Work out the finished part from the listing and answer in its coordinate system (mm). A direction names the side the tool comes from. Give positions to 0.01 mm unless a question says otherwise; leave off trailing zeros. Loops run counter-clockwise (first coordinate to the right, second up) from the corner with the lowest first, then second, coordinate; pieces in that order, holes last. Notation, with made-up numbers: M -1,41 L 20,41 A31 cw 20,73 Z; hole C -37,50.25 d7. An arc over 180 degrees is marked long. Answer as a JSON object with one key per item and string values. Group by question number.
```python
from build123d import *

# Parameters (mm, degrees)
SKETCH_1_R      = 1.5
EXTRUDE_1_DEPTH = 1.5
SKETCH_2_W      = 10
SKETCH_2_H      = 7.5
EXTRUDE_2_DEPTH = 10
SKETCH_3_W      = 8
SKETCH_3_H      = 8
EXTRUDE_3_DEPTH = 8
SKETCH_4_W      = 15
SKETCH_4_H      = 7.5
EXTRUDE_4_DEPTH = 10
EXTRUDE_5_DEPTH = 25
SKETCH_6_W      = 4
SKETCH_6_H      = 4
EXTRUDE_6_DEPTH = 4
SKETCH_7_W      = 20
SKETCH_7_H      = 5
EXTRUDE_7_DEPTH = 14
SKETCH_8_W      = 12
SKETCH_8_H      = 12
SKETCH_8_W_2    = 10
SKETCH_8_H_2    = 8
EXTRUDE_8_DEPTH = 8
SKETCH_9_R      = 4
EXTRUDE_9_DEPTH = 10


with BuildPart() as part:
    # 草图1 → 凸台-拉伸1 (new body)
    with BuildSketch(Plane(origin=(0, 0, 0), x_dir=(1, 0, 0), z_dir=(0, 1, 0))):
        with BuildLine():
            Line((-41.7, 30), (41.7, 30))
            ThreePointArc((41.7, 30), (44.033452378, 29.033452378), (45, 26.7))
            Line((45, 26.7), (45, -26.7))
            ThreePointArc((45, -26.7), (44.033452378, -29.033452378), (41.7, -30))
            Line((41.7, -30), (-41.7, -30))
            ThreePointArc((-41.7, -30), (-44.033452378, -29.033452378), (-45, -26.7))
            Line((-45, -26.7), (-45, 26.7))
            ThreePointArc((-45, 26.7), (-44.033452378, 29.033452378), (-41.7, 30))
        make_face()
        with Locations((-41.35, 26.4)):
            Circle(SKETCH_1_R, mode=Mode.SUBTRACT)
        with Locations((41.35, 26.4)):
            Circle(SKETCH_1_R, mode=Mode.SUBTRACT)
        with Locations((41.35, -26.4)):
            Circle(SKETCH_1_R, mode=Mode.SUBTRACT)
        with Locations((-41.35, -26.4)):
            Circle(SKETCH_1_R, mode=Mode.SUBTRACT)
    extrude(amount=EXTRUDE_1_DEPTH)

    # 草图2 → 凸台-拉伸2 (add)
    with BuildSketch(Plane(origin=(0, 1.5, 0), x_dir=(1, 0, 0), z_dir=(0, 1, 0))):
        with Locations((18.5, -23.75)):
            Rectangle(SKETCH_2_W, SKETCH_2_H)
        with Locations((-9.5, 23.75)):
            Rectangle(SKETCH_2_W, SKETCH_2_H)
        with Locations((9.5, 23.75)):
            Rectangle(SKETCH_2_W, SKETCH_2_H)
        with Locations((-18.5, -23.75)):
            Rectangle(SKETCH_2_W, SKETCH_2_H)
    extrude(amount=EXTRUDE_2_DEPTH)

    # 草图3 → 凸台-拉伸3 (add)
    with BuildSketch(Plane(origin=(0, 1.5, 0), x_dir=(1, 0, 0), z_dir=(0, 1, 0))):
        with Locations((-8.2, -23.75)):
            Rectangle(SKETCH_3_W, SKETCH_3_H)
    extrude(amount=EXTRUDE_3_DEPTH)

    # 草图4 → 凸台-拉伸4 (add)
    with BuildSketch(Plane(origin=(0, 1.5, 0), x_dir=(1, 0, 0), z_dir=(0, 1, 0))):
        with Locations((4.7, -23.75)):
            Rectangle(SKETCH_4_W, SKETCH_4_H)
    extrude(amount=EXTRUDE_4_DEPTH)

    # 草图5 → 凸台-拉伸5 (add)
    with BuildSketch(Plane(origin=(0, 1.5, 0), x_dir=(1, 0, 0), z_dir=(0, 1, 0))):
        Polygon((44.8, 16), (28.8, 16), (28.8, 15.4), (36.2, 15.4), (36.2, -6.4), (28.8, -6.4), (28.8, -7), (44.8, -7), (44.8, -6.4), (36.8, -6.4), (36.8, -2.52), (44.8, -2.52), (44.8, -1.92), (36.8, -1.92), (36.8, 1.96), (44.8, 1.96), (44.8, 2.56), (36.8, 2.56), (36.8, 6.44), (44.8, 6.44), (44.8, 7.04), (36.8, 7.04), (36.8, 10.92), (44.8, 10.92), (44.8, 11.52), (36.8, 11.52), (36.8, 15.4), (44.8, 15.4), align=None)
        Polygon((-44.8, 15.4), (-44.8, 16), (-28.8, 16), (-28.8, 15.4), (-36.2, 15.4), (-36.2, -6.4), (-28.8, -6.4), (-28.8, -7), (-44.8, -7), (-44.8, -6.4), (-36.8, -6.4), (-36.8, -2.52), (-44.8, -2.52), (-44.8, -1.92), (-36.8, -1.92), (-36.8, 1.96), (-44.8, 1.96), (-44.8, 2.56), (-36.8, 2.56), (-36.8, 6.44), (-44.8, 6.44), (-44.8, 7.04), (-36.8, 7.04), (-36.8, 10.92), (-44.8, 10.92), (-44.8, 11.52), (-36.8, 11.52), (-36.8, 15.4), align=None)
    extrude(amount=EXTRUDE_5_DEPTH)

    # 草图6 → 凸台-拉伸6 (add)
    with BuildSketch(Plane(origin=(0, 9.5, 0), x_dir=(1, 0, 0), z_dir=(0, 1, 0))):
        with Locations((-8.2, -23.75)):
            Rectangle(SKETCH_6_W, SKETCH_6_H)
    extrude(amount=EXTRUDE_6_DEPTH)

    # 草图7 → 凸台-拉伸7 (add)
    with BuildSketch(Plane(origin=(0, 1.5, 0), x_dir=(1, 0, 0), z_dir=(0, 1, 0))):
        with Locations((0, 10.5)):
            Rectangle(SKETCH_7_W, SKETCH_7_H)
    extrude(amount=EXTRUDE_7_DEPTH)

    # 草图8 → 凸台-拉伸8 (add)
    with BuildSketch(Plane(origin=(0, 1.5, 0), x_dir=(1, 0, 0), z_dir=(0, 1, 0))):
        with Locations((8.02497304, -3.633209752)):
            Rectangle(SKETCH_8_W, SKETCH_8_H)
        with Locations((-7.684380811, -4.555618829)):
            Rectangle(SKETCH_8_W_2, SKETCH_8_H_2)
    extrude(amount=EXTRUDE_8_DEPTH)

    # 草图9 → 凸台-拉伸9 (add)
    with BuildSketch(Plane(origin=(0, 1.5, 0), x_dir=(1, 0, 0), z_dir=(0, 1, 0))):
        with Locations((-19, 1.275195949)):
            Circle(SKETCH_9_R)
        with Locations((19, -1.275195949)):
            Circle(SKETCH_9_R)
    extrude(amount=EXTRUDE_9_DEPTH)


solid = part.part
```
Item 1: A cutting plane is placed at A-A (x = 19). Determine the outline of the cut face in (y, z), and give its area (3 significant figures).
Item 2: A tool of negligible diameter and unlimited length cuts with its end or side. For faces 4 (the flat face through (-8, 5, 0.556)), 5 (the flat face through (-37, 14, 7)), 6 (the flat face through (-8, 13.5, 24)), 7 (the flat face through (37, 14, 7)), 8 (the flat face through (41, 14, -10.92)), from which of +Z, -Z, +X, -X, +Y, -Y can it reach the whole face along a straight path? Write none if from no direction.
Item 3: A cutting plane is placed at B-B (z = -22). Determine the outline of the cut face in (x, y).
Item 4: A cutting plane is placed at C-C (x = 8). Determine the outline of the cut face in (y, z), and give its area (3 significant figures).
Item 5: For a pull along X with two mould halves and no side action, classify faces 1 (the flat face through (-4.5, 6, -24)), 2 (the flat face through (-41, 14, 2.52)), 3 (the flat face through (23.5, 6, 24)) as pulls with the +X half, pulls with the -X half, needs draft (parallel to the pull), parting line crosses it, or undercut.
Item 6: Given pin 1 Ø4 at (x, y) = (-7, 4.5) entering from +Z; pin 2 Ø9 at (x, y) = (41.5, 15) entering from -Z; pin 3 Ø6.5 at (x, y) = (-42.5, 14.5) entering from +Z, each flat-ended and moving along its own axis, determine where each tip first touches the part or whether it passes through.
Item 7: Find the intervals of material crossed by probe 1 along Z at (x, y) = (41.35, 0.3); probe 2 along X at (y, z) = (0.7, -26.4); probe 3 along X at (y, z) = (8, -10), in increasing order. Write a range as [from, to].
The answers:
{
 "1": {"outline": "M 0,-30 L 1.5,-30 L 1.5,-2.72 L 11.5,-2.72 L 11.5,5.28 L 1.5,5.28 L 1.5,20 L 11.5,20 L 11.5,27.5 L 1.5,27.5 L 1.5,30 L 0,30 Z", "area": "245 mm^2"},
 "2": {"face 4": "+Y", "face 5": "+Z, -X, +Y", "face 6": "+Z, +X, -X, +Y", "face 7": "+Z, +X, +Y", "face 8": "+X, +Y"},
 "3": {"outline": "M -45,0 L 45,0 L 45,1.5 L 14.5,1.5 L 14.5,11.5 L 4.5,11.5 L 4.5,1.5 L -4.5,1.5 L -4.5,11.5 L -14.5,11.5 L -14.5,1.5 L -45,1.5 Z"},
 "4": {"outline": "M 0,-30 L 1.5,-30 L 1.5,-27.5 L 11.5,-27.5 L 11.5,-20 L 1.5,-20 L 1.5,-13 L 15.5,-13 L 15.5,-8 L 1.5,-8 L 1.5,-2.37 L 9.5,-2.37 L 9.5,9.63 L 1.5,9.63 L 1.5,20 L 11.5,20 L 11.5,27.5 L 1.5,27.5 L 1.5,30 L 0,30 Z", "area": "406 mm^2"},
 "5": {"face 1": "undercut", "face 2": "needs draft", "face 3": "pulls with the +X half"},
 "6": {"pin 1": "stops at z = 27.75", "pin 2": "stops at z = -16", "pin 3": "stops at z = 7"},
 "7": {"probe 1": "z = [-30, -27.9], [-24.9, 24.9], [27.9, 30]", "probe 2": "x = [-45, -42.85], [-39.85, 39.85], [42.85, 45]", "probe 3": "x = [-36.8, -36.2], [-10, 10], [36.2, 36.8]"}
}
